Work out the finished part from the listing and answer in its coordinate system (mm). A direction names the side the tool comes from. Give positions to 0.01 mm unless a question says otherwise; leave off trailing zeros. Write each loop counter-clockwise with the first axis right and the second up, starting at its lowest first coordinate (ties: lowest second). Pieces come first, ordered by that corner, then holes. Notation, with made-up numbers: (-6.5, 66) -> (4.5, 66) arc R18 cw to (4.5, 93) -> close; hole circle Ø7 at (81.25, 1). An arc over 180 degrees is marked (long way). Use a Markdown table: item, result. Add a question column.
Q1. Each of these flat-tipped pins is pushed along its axis until it touches: pin 1 Ø1.5 at (x, y) = (-42, 23.5) entering from +Z; pin 2 Ø5 at (y, z) = (24, 0) entering from -X; pin 3 Ø10 at (x, z) = (-51, 32.5) entering from -Y. Where does it stop, or does it pass through?
Q2. Section B-B, the plane z = 37 is taken. Give the vertices of the cut face in (x, y), plus the area to 3 significant figures.
Q3. Section A-A, the plane z = -1 is taken. Give the vertices of the cut face in (x, y).
Q4. For faces 1 (the face through (-47.726, 10.977, 36.853)), 2 (the face through (-45, 11, 47.5)), determine the directions among +Z, -Z, +X, -X, +Y, -Y from which every point of the face is accessible in a straight line to the end or side of a thin tool.
Q5. Consider line 1 (Y direction, x = -45, z = 36.5); line 2 (Z direction, x = -42, y = 15.5); line 3 (Z direction, x = -42, y = 26.5). Determine where each line is inside the solid, lowest interval first.
from build123d import *

# Parameters (mm, degrees)
F0_R     = 18.5
F1_DEPTH = 16
F2_R     = 18.5
F3_DEPTH = 10.5
F4_SIZE2 = 10.5
F4_SIZE  = 10.5
F5_R     = 18.5
F6_DEPTH = 10.5
F7_SIZE2 = 10.5
F7_SIZE  = 10.5
F8_R     = 2.5
F9_DEPTH = 21


with BuildPart() as f1:
    # F0 (on Top) → F1 (new body)
    with BuildSketch(Plane.XY):
        with Locations((-45.2287606895, 10.8666494489)):
            Circle(F0_R)
    extrude(amount=F1_DEPTH)

    # F2 (on face) → F3 (join)
    with BuildSketch(Plane(origin=(0, 0, 0), x_dir=(1, 0, 0), z_dir=(0, 0, -1))):
        with Locations((-45.2287606895, -10.8666494489)):
            Circle(F2_R)
    extrude(amount=F3_DEPTH)

    # F4
    f4_edges = [f1.edges().sort_by_distance(p)[0] for p in [
        (-63.728761, 10.866649, -10.5),
    ]]
    chamfer(f4_edges, length=F4_SIZE, length2=F4_SIZE2)

    # F5 (on face) → F6 (join)
    with BuildSketch(Plane.XY.offset(16)):
        with Locations((-45.2287606895, 10.8666494489)):
            Circle(F5_R)
    extrude(amount=F6_DEPTH)

    # F7
    f7_edges = [f1.edges().sort_by_distance(p)[0] for p in [
        (-63.728761, 10.866649, 26.5),
    ]]
    chamfer(f7_edges, length=F7_SIZE, length2=F7_SIZE2)

    # F8 (on face) → F9 (join)
    with BuildSketch(Plane.XY.offset(26.5)):
        with Locations((-45.2287606895, 10.8666494489)):
            Circle(F8_R)
    extrude(amount=F9_DEPTH)


solid = f1.part
Result set:
| question | item | result |
|---|---|---|
| 1 | pin 1 | stops at z = 22.21 |
| 1 | pin 2 | stops at x = -60.37 |
| 1 | pin 3 | stops at y = 8.49 |
| 2 | outline | circle Ø5 at (-45.23, 10.87) |
| 2 | area | 19.6 mm2 |
| 3 | outline | circle Ø35 at (-45.23, 10.87) |
| 4 | face 1 | +Z |
| 4 | face 2 | +Z, +X, -X, +Y, -Y |
| 5 | line 1 | y = 8.38 to 13.36 |
| 5 | line 2 | z = -10.5 to 26.5 |
| 5 | line 3 | z = -2.54 to 18.54 |
